```python
from build123d import *

# Parameters (mm, degrees)
HOLE_WIZARD_M3_1_D = 2.5


with BuildPart() as part:
    # 草图1 → 旋转1 (revolve)
    with BuildSketch(Plane.XY, mode=Mode.PRIVATE) as revolve_1_sk:
        Polygon((1.5, 0), (9.85, 0), (9.85, -2.3), (4.4, -2.3), (4.4, -4.3), (3, -4.3), (3, -0.8), (1.5, -0.8), align=None)
    revolve(revolve_1_sk.sketch.rotate(Axis((0, 0, 0), (0, 1, 0)), 90), axis=Axis((0, 0, 0), (0, 1, 0)))

    # M3 螺纹孔1 (through all)
    with Locations(Plane(origin=(0, 0, 0), x_dir=(1, 0, 0), z_dir=(0, 1, 0))):
        with Locations((0, 6.75), (6.75, 0), (0, -6.75), (-6.75, 0)):
            Hole(HOLE_WIZARD_M3_1_D / 2)


solid = part.part
```
Part model, mm, in its own coordinate system. A direction names the side the tool comes from. Give positions to 0.01 mm unless a question says otherwise; leave off trailing zeros. Order: outer loops, then holes, each group sorted by start corner. A loop starts at its lowest first (then second) coordinate and runs counter-clockwise, first axis right, second up. Notation, with made-up numbers: (83, 0.25) - (101, 0.25) arc R27 cw to (101, 26.25) - close; hole circle Ø3 at (75.25, 2.5). An arc over 180 degrees is marked (long way). Use one line per item in the form item = value.
Item 1: Slice it at B-B on z = 0. Give the cut face in (x, y), and give its area (3 significant figures).
Solution:
outline = (-9.85, -2.3) - (-8, -2.3) - (-8, 0) - (-9.85, 0) - close; (-5.5, -2.3) - (-4.4, -2.3) - (-4.4, -4.3) - (-3, -4.3) - (-3, -0.8) - (-1.5, -0.8) - (-1.5, 0) - (-5.5, 0) - close; (1.5, -0.8) - (3, -0.8) - (3, -4.3) - (4.4, -4.3) - (4.4, -2.3) - (5.5, -2.3) - (5.5, 0) - (1.5, 0) - close; (8, -2.3) - (9.85, -2.3) - (9.85, 0) - (8, 0) - close
area = 28.0 mm2
Item 2: Probe probe 1 along X at (y, z) = (-3.05, 0); probe 2 along Y at (x, z) = (-4.5, -3); probe 3 along X at (y, z) = (-1.8, -1.75). List the from-to ranges inside material, lowest first. Write a range as from..to.
Solution:
probe_1 = -4.4..-3, 3..4.4
probe_2 = -2.3..0
probe_3 = -9.69..-2.44, 2.44..9.69
Item 3: Which spindle directions (+Z, -Z, +X, -X, +Y, -Y) get a long thin tool onto all of the face, cutting with end or side? Do faces 4 (the face through (0.27, -1.17, -5.53)), 5 (the face through (1.3, -0.8, -1.3)). Say none if no direction does.
Solution:
face_4 = +Y, -Y
face_5 = -Y
Item 4: Slice it at A-A on x = 0. Give the cut face in (y, z), and give its area (3 significant figures).
Solution:
outline = (-4.3, -4.4) - (-2.3, -4.4) - (-2.3, -5.5) - (0, -5.5) - (0, -1.5) - (-0.8, -1.5) - (-0.8, -3) - (-4.3, -3) - close; (-4.3, 3) - (-0.8, 3) - (-0.8, 1.5) - (0, 1.5) - (0, 5.5) - (-2.3, 5.5) - (-2.3, 4.4) - (-4.3, 4.4) - close; (-2.3, -9.85) - (0, -9.85) - (0, -8) - (-2.3, -8) - close; (-2.3, 8) - (0, 8) - (0, 9.85) - (-2.3, 9.85) - close
area = 28.0 mm2
Item 5: Slice it at D-D on z = 7.25. Give the cut face in (x, y), and give its area (3 significant figures).
Solution:
outline = (-6.67, -2.3) - (-1.15, -2.3) - (-1.15, 0) - (-6.67, 0) - close; (1.15, -2.3) - (6.67, -2.3) - (6.67, 0) - (1.15, 0) - close
area = 25.4 mm2
Item 6: Two-plate mould, pull along X, no slides. Class faces 1 (the face through (4.2, -2.3, -2.1)), 2 (the face through (5.99, -1.17, 7.82)), 3 (the face through (-0.45, -0.39, -1.43)): released by +X, released by -X, zero draft, split by the parting line, or undercut.
Solution:
face_1 = zero draft
face_2 = split by the parting line
face_3 = undercut
Item 7: Slice it at C-C on x = -6. Give the cut face in (y, z).
Solution:
outline = (-2.3, -7.81) - (0, -7.81) - (0, -1) - (-2.3, -1) - close; (-2.3, 1) - (0, 1) - (0, 7.81) - (-2.3, 7.81) - close
Item 8: Pin check, flat tips, straight feed: pin 1 Ø1 at (x, y) = (-2, -3.5) entering from +Z; pin 2 Ø4 at (x, z) = (0, -6.75) entering from -Y; pin 3 Ø4 at (x, z) = (0, 0) entering from -Y. Stop position of each tip, or through.
Solution:
pin_1 = 4.14
pin_2 = -2.3
pin_3 = -0.8
